Build history of the part. All positions in model axes, mm. A direction names the side the tool comes from. Round coordinates to 2 decimals unless told otherwise and drop trailing zeros. Write each loop counter-clockwise with the first axis right and the second up, starting at its lowest first coordinate (ties: lowest second). Pieces come first, ordered by that corner, then holes.
1) Saw through at B-B (z = -56.5). Write the cut outline in (x, y).
2) Which spindle directions (+Z, -Z, +X, -X, +Y, -Y) get a long thin tool onto all of the face, cutting with end or side? Do faces 1 (the flat face through (70, 15, -35)), 2 (the flat face through (70, 15, -25)), 3 (the flat face through (70, 15, -55)), 4 (the cylindrical face through (5.07, 15.526, -51.669)), 5 (the flat face through (82, 5, -70)). Say none if no direction does.
3) Saw through at A-A (x = 41.5). Write the cut outline in (y, z).
4) Wall check: probe 1 along X at (y, z) = (1, -50.5); probe 2 along Y at (x, z) = (93.8, -49); probe 3 along Y at (x, z) = (70, -30). Give the ranges that are in metal, low to high.
5) Saw through at C-C (y = 2). Write the cut outline in (x, z), plus the area to 3 significant figures.
6) Pull direction Y, two halves, no side cores. Call faces 6 (the flat face through (47, 5, 0)), 7 (the cylindrical face through (70.03, 16.18, -28.71)), 8 (the flat face through (70, 20, -30)): +Y half, -Y half, draft (parallel to the pull), parting line (faces both ways), or undercut.
7) Flat gauge pins, fed straight in: pin 1 (3 mm diameter, centred on x = 6, z = -37.5, fed in from +Y); pin 2 (2 mm diameter, centred on x = 70, y = 14.5, fed in from +Z); pin 3 (6 mm diameter, centred on x = 47, z = -14.5, fed in from -Y); pin 4 (2 mm diameter, centred on x = 71, y = 16, fed in from -Z). Where does each tip first touch, or does it go through?
from build123d import *

# Parameters (mm, degrees)
SKETCH1_W           = 96
SKETCH1_H           = 80
SKETCH1_W_2         = 82
SKETCH1_H_2         = 60
BOSS_EXTRUDE1_DEPTH = 10
BOSS_EXTRUDE2_REACH = 121.231
SKETCH5_W           = 4
SKETCH5_H           = 10
SKETCH6_W           = 10
SKETCH6_H           = 10
SKETCH6_W_2         = 4
BOSS_EXTRUDE3_DEPTH = 10
SKETCH7_R           = 1.75
CUT_EXTRUDE3_DEPTH  = 110.471457467
CUT_EXTRUDE4_REACH  = 128.554
SKETCH10_R          = 1.75


with BuildPart() as part:
    # Sketch1 → Boss-Extrude1 (new body)
    with BuildSketch(Plane(origin=(0, 0, 0), x_dir=(1, 0, 0), z_dir=(0, 1, 0))):
        with Locations((48, 40)):
            Rectangle(SKETCH1_W, SKETCH1_H)
        with Locations((51, 40)):
            Rectangle(SKETCH1_W_2, SKETCH1_H_2, mode=Mode.SUBTRACT)
    extrude(amount=BOSS_EXTRUDE1_DEPTH)

    # Sketch5 → Boss-Extrude2 (add, up to next)
    with BuildSketch(Plane.XY.offset(-70), mode=Mode.PRIVATE) as boss_extrude2_sk1:
        with Locations((70, 5)):
            Rectangle(SKETCH5_W, SKETCH5_H)
    boss_extrude2_tool1 = extrude(boss_extrude2_sk1.sketch, amount=BOSS_EXTRUDE2_REACH, mode=Mode.PRIVATE) - part.part
    add(boss_extrude2_tool1.solids().sort_by_distance((70, 5, -70))[0])

    # Sketch6 → Boss-Extrude3 (add)
    with BuildSketch(Plane(origin=(0, 10, 0), x_dir=(1, 0, 0), z_dir=(0, 1, 0))):
        with Locations((5, 50)):
            Rectangle(SKETCH6_W, SKETCH6_H)
        with Locations((5, 30)):
            Rectangle(SKETCH6_W, SKETCH6_H)
        with Locations((70, 50)):
            Rectangle(SKETCH6_W_2, SKETCH6_H)
        with Locations((70, 30)):
            Rectangle(SKETCH6_W_2, SKETCH6_H)
    extrude(amount=BOSS_EXTRUDE3_DEPTH)

    # Sketch7 → Cut-Extrude3 (cut, through all)
    with BuildSketch(Plane(origin=(72, 0, 0), x_dir=(0, 0, -1), z_dir=(1, 0, 0))):
        with Locations((30, 15)):
            Circle(SKETCH7_R)
        with Locations((50, 15)):
            Circle(SKETCH7_R)
    extrude(amount=-CUT_EXTRUDE3_DEPTH, mode=Mode.SUBTRACT)

    # Sketch10 → Cut-Extrude4 (cut, up to next)
    with BuildSketch(Plane(origin=(96, 0, 0), x_dir=(0, 0, -1), z_dir=(1, 0, 0)), mode=Mode.PRIVATE) as cut_extrude4_sk1:
        with Locations((31, 5)):
            Circle(SKETCH10_R)
    cut_extrude4_tool1 = extrude(cut_extrude4_sk1.sketch, amount=-CUT_EXTRUDE4_REACH, mode=Mode.PRIVATE) & part.part
    # Sketch10 → Cut-Extrude4 (cut, up to next)
    with BuildSketch(Plane(origin=(96, 0, 0), x_dir=(0, 0, -1), z_dir=(1, 0, 0)), mode=Mode.PRIVATE) as cut_extrude4_sk2:
        with Locations((49, 5)):
            Circle(SKETCH10_R)
    cut_extrude4_tool2 = extrude(cut_extrude4_sk2.sketch, amount=-CUT_EXTRUDE4_REACH, mode=Mode.PRIVATE) & part.part
    add(cut_extrude4_tool1.solids().sort_by_distance((96, 5, -31))[0], mode=Mode.SUBTRACT)
    add(cut_extrude4_tool2.solids().sort_by_distance((96, 5, -49))[0], mode=Mode.SUBTRACT)


solid = part.part
Evaluation:
1. outline: (0, 0) - (10, 0) - (10, 10) - (0, 10) - close; (68, 0) - (72, 0) - (72, 10) - (68, 10) - close; (92, 0) - (96, 0) - (96, 10) - (92, 10) - close
2. face 1: +X, -X, +Y
2. face 2: +Z, +X, -X, +Y
2. face 3: -Z, +X, -X, +Y
2. face 4: +X, -X
2. face 5: +Y, -Y
3. outline: (0, -80) - (10, -80) - (10, -70) - (0, -70) - close; (0, -10) - (10, -10) - (10, 0) - (0, 0) - close
4. probe 1: x = 0 to 10, 68 to 72, 92 to 96
4. probe 2: y = 0 to 3.25, 6.75 to 10
4. probe 3: y = 0 to 13.25, 16.75 to 20
5. outline: (0, -80) - (96, -80) - (96, 0) - (0, 0) - close; hole (10, -70) - (68, -70) - (68, -10) - (10, -10) - close; hole (72, -70) - (92, -70) - (92, -10) - (72, -10) - close
5. area: 3,000 mm2
6. face 6: draft
6. face 7: undercut
6. face 8: +Y half
7. pin 1: stops at y = 10
7. pin 2: stops at z = -25
7. pin 3: passes through
7. pin 4: stops at z = -55
